The listing builds one solid part. Answer for the finished solid, in the listing's coordinates (mm). Round coordinates to 2 decimals unless told otherwise and drop trailing zeros. Loops run counter-clockwise (first coordinate to the right, second up) from the corner with the lowest first, then second, coordinate; pieces in that order, holes last. Notation, with made-up numbers: (81, 57.5) -> (85, 57.5) arc R20 ccw to (85, 78.5) -> close; hole circle Ø1 at (20, 61). An arc over 180 degrees is marked (long way). Use a Markdown table: item, result. Add a question column.
Q1. Consider line 1 (Y direction, x = -7.4, z = 2.55); line 2 (X direction, y = -67, z = 3.95); line 3 (Y direction, x = -2.5, z = 1.55). Determine where each line is inside the solid, lowest interval first.
Q2. Given pin 1 Ø8 at (x, y) = (-7.4, 42.6) entering from -Z; pin 2 Ø1.5 at (x, z) = (-1.5, 1.5) entering from +Y, each flat-ended and moving along its own axis, determine where each tip first touches the part or whether it passes through.
Q3. Section B-B on y = 23 is taken. Give the vertices of the cut face in (x, z).
Q4. Section A-A on z = 3.3 is taken. Give the number of separate pieces and of enclosed holes in the cut face, then the cut area to 3 significant figures.
Q5. Section C-C on x = 20 is taken. Give the vertices of the cut face in (y, z), then the cut area to 4 significant figures.
from build123d import *

# Parameters (mm, degrees)
SKETCH2_W               = 255
SKETCH2_H               = 250
BOSS_EXTRUDE1_DEPTH     = 5
SKETCH4_W               = 20
SKETCH4_H               = 54.5
CUT_EXTRUDE1_DEPTH      = 32
CUT_EXTRUDE1_DEPTH_BACK = 23
SKETCH5_W               = 20
SKETCH5_H               = 7.25
BOSS_EXTRUDE3_DEPTH     = 5
CUT_EXTRUDE2_DEPTH      = 23
SKETCH7_R               = 2.5
CUT_EXTRUDE3_DEPTH      = 23
BOSS_EXTRUDE6_DEPTH     = 5
SKETCH9_W               = 0.5
SKETCH9_H               = 0.5
BOSS_EXTRUDE7_DEPTH     = 5
SKETCH10_W              = 6
SKETCH10_H              = 65
BOSS_EXTRUDE8_DEPTH     = 5
SKETCH10_3_W            = 5
SKETCH10_3_H            = 30
CUT_EXTRUDE4_DEPTH      = 10
SKETCH11_W              = 6
SKETCH11_H              = 185
BOSS_EXTRUDE9_DEPTH     = 5
SKETCH14_W              = 6
SKETCH14_H              = 250
CUT_EXTRUDE5_DEPTH      = 10
CUT_EXTRUDE6_DEPTH      = 185
SKETCH16_R              = 1.5
CUT_EXTRUDE7_DEPTH      = 185
SKETCH17_R              = 1.5
CUT_EXTRUDE8_DEPTH      = 185
SKETCH18_R              = 2
CUT_EXTRUDE9_DEPTH      = 10


with BuildPart() as part:
    # Sketch2 → Boss-Extrude1 (new body)
    with BuildSketch(Plane.XY):
        with Locations((-2.5, 0)):
            Rectangle(SKETCH2_W, SKETCH2_H)
    extrude(amount=BOSS_EXTRUDE1_DEPTH)

    # Sketch4 → Cut-Extrude1 (cut, two sides)
    with BuildSketch(Plane(origin=(0, 0, 0), x_dir=(-1, 0, 0), z_dir=(0, 0, -1))) as cut_extrude1_sk:
        with Locations((2.5, 18.3)):
            Rectangle(SKETCH4_W, SKETCH4_H)
    extrude(amount=CUT_EXTRUDE1_DEPTH, mode=Mode.SUBTRACT)
    extrude(cut_extrude1_sk.sketch, amount=-CUT_EXTRUDE1_DEPTH_BACK, mode=Mode.SUBTRACT)

    # Sketch5 → Boss-Extrude3 (add)
    with BuildSketch(Plane(origin=(0, 0, 0), x_dir=(-1, 0, 0), z_dir=(0, 0, -1))):
        with Locations((2.5, 41.925)):
            Rectangle(SKETCH5_W, SKETCH5_H)
        with Locations((2.5, -5.325)):
            Rectangle(SKETCH5_W, SKETCH5_H)
    extrude(amount=-BOSS_EXTRUDE3_DEPTH)

    # Sketch6 → Cut-Extrude2 (cut)
    with BuildSketch(Plane(origin=(0, 0, 0), x_dir=(-1, 0, 0), z_dir=(0, 0, -1))):
        Polygon((-7.5, 38.3), (-7.5, 48.3), (-32.5, 48.3), (-32.5, -11.7), (-7.5, -11.7), (-7.5, -1.7), align=None)
    extrude(amount=-CUT_EXTRUDE2_DEPTH, mode=Mode.SUBTRACT)

    # Sketch7 → Cut-Extrude3 (cut)
    with BuildSketch(Plane(origin=(0, 0, 0), x_dir=(-1, 0, 0), z_dir=(0, 0, -1))):
        with Locations((-2.4, 42.6)):
            Circle(SKETCH7_R)
        with Locations((7.4, 42.6)):
            Circle(SKETCH7_R)
        with Locations((-2.4, -6)):
            Circle(SKETCH7_R)
        with Locations((7.4, -6)):
            Circle(SKETCH7_R)
    extrude(amount=-CUT_EXTRUDE3_DEPTH, mode=Mode.SUBTRACT)

    # Sketch8 → Boss-Extrude6 (add)
    with BuildSketch(Plane(origin=(0, 0, 0), x_dir=(-1, 0, 0), z_dir=(0, 0, -1))):
        Polygon((-8, 38.8), (-7.5, 38.8), (-7.5, 48.3), (-32.5, 48.3), (-32.5, -11.7), (-7.5, -11.7), (-7.5, -2.2), (-8, -2.2), align=None)
    extrude(amount=-BOSS_EXTRUDE6_DEPTH)

    # Sketch9 → Boss-Extrude7 (add)
    with BuildSketch(Plane(origin=(0, 0, 0), x_dir=(-1, 0, 0), z_dir=(0, 0, -1))):
        with Locations((-7.75, 38.55)):
            Rectangle(SKETCH9_W, SKETCH9_H)
        with Locations((-7.75, -1.95)):
            Rectangle(SKETCH9_W, SKETCH9_H)
    extrude(amount=-BOSS_EXTRUDE7_DEPTH)

    # Sketch10 → Boss-Extrude8 (add)
    with BuildSketch(Plane(origin=(0, 0, 0), x_dir=(-1, 0, 0), z_dir=(0, 0, -1))):
        Polygon((130, -107.5), (130, -125), (136, -125), (136, -60), (130, -60), (130, -77.5), align=None)
        with Locations((-128, -92.5)):
            Rectangle(SKETCH10_W, SKETCH10_H)
    extrude(amount=-BOSS_EXTRUDE8_DEPTH)

    # Sketch10<3> → Cut-Extrude4 (cut)
    with BuildSketch(Plane(origin=(0, 0, 0), x_dir=(-1, 0, 0), z_dir=(0, 0, -1))):
        with Locations((127.5, -92.5)):
            Rectangle(SKETCH10_3_W, SKETCH10_3_H)
        with Locations((-122.5, -92.5)):
            Rectangle(SKETCH10_3_W, SKETCH10_3_H)
    extrude(amount=-CUT_EXTRUDE4_DEPTH, mode=Mode.SUBTRACT)

    # Sketch11 → Boss-Extrude9 (add)
    with BuildSketch(Plane(origin=(0, 0, 0), x_dir=(-1, 0, 0), z_dir=(0, 0, -1))):
        with Locations((-128, 32.5)):
            Rectangle(SKETCH11_W, SKETCH11_H)
        with Locations((133, 32.5)):
            Rectangle(SKETCH11_W, SKETCH11_H)
    extrude(amount=-BOSS_EXTRUDE9_DEPTH)

    # Sketch14 → Cut-Extrude5 (cut)
    with BuildSketch(Plane(origin=(0, 0, 0), x_dir=(-1, 0, 0), z_dir=(0, 0, -1))):
        with Locations((-128, 0)):
            Rectangle(SKETCH14_W, SKETCH14_H)
        with Locations((133, 0)):
            Rectangle(SKETCH14_W, SKETCH14_H)
    extrude(amount=-CUT_EXTRUDE5_DEPTH, mode=Mode.SUBTRACT)

    # Sketch15 → Cut-Extrude6 (cut)
    with BuildSketch(Plane(origin=(0, 0, 0), x_dir=(-1, 0, 0), z_dir=(0, 0, -1))):
        Polygon((2.5, 125), (-61.25, 125), (-61.25, 120), (2.5, 120), (66.25, 120), (66.25, 125), align=None)
    extrude(amount=-CUT_EXTRUDE6_DEPTH, mode=Mode.SUBTRACT)

    # Sketch16 → Cut-Extrude7 (cut)
    with BuildSketch(Plane(origin=(0, 0, 0), x_dir=(-1, 0, 0), z_dir=(0, 0, -1))):
        with Locations((-93.125, 110)):
            Circle(SKETCH16_R)
        with Locations((98.125, 110)):
            Circle(SKETCH16_R)
    extrude(amount=-CUT_EXTRUDE7_DEPTH, mode=Mode.SUBTRACT)

    # Sketch17 → Cut-Extrude8 (cut)
    with BuildSketch(Plane(origin=(0, 0, 0), x_dir=(-1, 0, 0), z_dir=(0, 0, -1))):
        with Locations((-110, -68.75)):
            Circle(SKETCH17_R)
        with Locations((115, -68.75)):
            Circle(SKETCH17_R)
    extrude(amount=-CUT_EXTRUDE8_DEPTH, mode=Mode.SUBTRACT)

    # Sketch18 → Cut-Extrude9 (cut)
    with BuildSketch(Plane(origin=(0, 0, 0), x_dir=(-1, 0, 0), z_dir=(0, 0, -1))):
        with Locations((-93.125, 110)):
            Circle(SKETCH18_R)
        with Locations((98.125, 110)):
            Circle(SKETCH18_R)
        with Locations((115, -68.75)):
            Circle(SKETCH18_R)
        with Locations((-110, -68.75)):
            Circle(SKETCH18_R)
    extrude(amount=-CUT_EXTRUDE9_DEPTH, mode=Mode.SUBTRACT)


solid = part.part
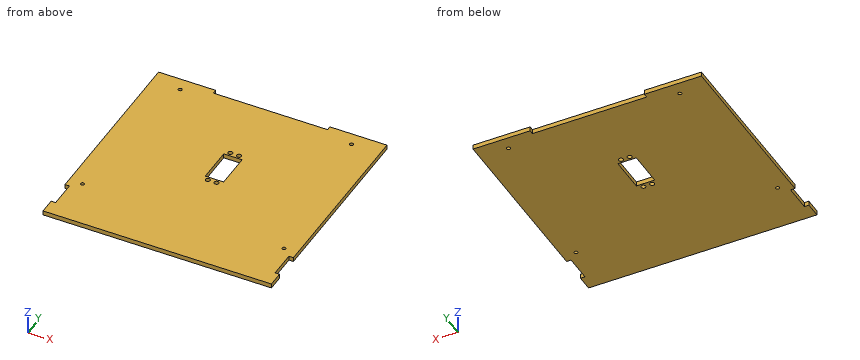
Checked values:
| question | item | result |
|---|---|---|
| 1 | line 1 | y = -125 to -8.5, -3.5 to -1.7, 38.3 to 40.1, 45.1 to 120 |
| 1 | line 2 | x = -130 to -115.97, -114.03 to 109.03, 110.97 to 125 |
| 1 | line 3 | y = -125 to -1.7, 38.3 to 120 |
| 2 | pin 1 | stops at z = 0 |
| 2 | pin 2 | stops at y = 120 |
| 3 | outline | (-130, 0) -> (-12.5, 0) -> (-12.5, 5) -> (-130, 5) -> close; (8, 0) -> (125, 0) -> (125, 5) -> (8, 5) -> close |
| 4 | separate pieces | 1 |
| 4 | enclosed holes | 9 |
| 4 | area | 61,900 mm2 |
| 5 | outline | (-125, 0) -> (120, 0) -> (120, 5) -> (-125, 5) -> close |
| 5 | area | 1,225 mm2 |
